Autodesk Inventor part; units mm, degrees
ref_plane "C1_XY" through (0, 0, 0) normal (0, 0, 1) x (1, 0, 0)
ref_plane "C1_YZ" through (0, 0, 0) normal (1, 0, 0) x (0, 1, 0)
ref_plane "C1_ZX" through (0, 0, 0) normal (0, 1, 0) x (0, 0, 1)
sketch "Sketch_1" plane through (0, 0, 0) normal (0, 0, 1) x (1, 0, 0)
  line L0 (-15, -4) -> (-15, -13)
  arc A0 (-15, -13) -> (-13, -15) centre (-13, -13) ccw
  line L1 (-13, -15) -> (-4, -15)
  line L2 (-4, -15) -> (-4, -13)
  line L3 (-4, -13) -> (-8.25, -13)
  line L4 (-8.25, -13) -> (-8.25, -9.6642)
  line L5 (-8.25, -9.6642) -> (-4.5858, -6)
  line L6 (-4.5858, -6) -> (-0.5196, -6)
  line L7 (-0.5196, -6) -> (0, -5.7)
  line L8 (0, -5.7) -> (0.5196, -6)
  line L9 (0.5196, -6) -> (4.5858, -6)
  line L10 (4.5858, -6) -> (8.25, -9.6642)
  line L11 (8.25, -9.6642) -> (8.25, -13)
  line L12 (8.25, -13) -> (4, -13)
  line L13 (4, -13) -> (4, -15)
  line L14 (4, -15) -> (13, -15)
  arc A1 (13, -15) -> (15, -13) centre (13, -13) ccw
  line L15 (15, -13) -> (15, -4)
  line L16 (15, -4) -> (13, -4)
  line L17 (13, -4) -> (13, -8.25)
  line L18 (13, -8.25) -> (9.6642, -8.25)
  line L19 (9.6642, -8.25) -> (6, -4.5858)
  line L20 (6, -4.5858) -> (6, -0.5196)
  line L21 (6, -0.5196) -> (5.7, 0)
  line L22 (5.7, 0) -> (6, 0.5196)
  line L23 (6, 0.5196) -> (6, 4.5858)
  line L24 (6, 4.5858) -> (9.6642, 8.25)
  line L25 (9.6642, 8.25) -> (13, 8.25)
  line L26 (13, 8.25) -> (13, 4)
  line L27 (13, 4) -> (15, 4)
  line L28 (15, 4) -> (15, 13)
  arc A2 (15, 13) -> (13, 15) centre (13, 13) ccw
  line L29 (13, 15) -> (4, 15)
  line L30 (4, 15) -> (4, 13)
  line L31 (4, 13) -> (8.25, 13)
  line L32 (8.25, 13) -> (8.25, 9.6642)
  line L33 (8.25, 9.6642) -> (4.5858, 6)
  line L34 (4.5858, 6) -> (0.5196, 6)
  line L35 (0.5196, 6) -> (0, 5.7)
  line L36 (0, 5.7) -> (-0.5196, 6)
  line L37 (-0.5196, 6) -> (-4.5858, 6)
  line L38 (-4.5858, 6) -> (-8.25, 9.6642)
  line L39 (-8.25, 9.6642) -> (-8.25, 13)
  line L40 (-8.25, 13) -> (-4, 13)
  line L41 (-4, 13) -> (-4, 15)
  line L42 (-4, 15) -> (-13, 15)
  arc A3 (-13, 15) -> (-15, 13) centre (-13, 13) ccw
  line L43 (-15, 13) -> (-15, 4)
  line L44 (-15, 4) -> (-13, 4)
  line L45 (-13, 4) -> (-13, 8.25)
  line L46 (-13, 8.25) -> (-9.6642, 8.25)
  line L47 (-9.6642, 8.25) -> (-6, 4.5858)
  line L48 (-6, 4.5858) -> (-6, 0.5196)
  line L49 (-6, 0.5196) -> (-5.7, 0)
  line L50 (-5.7, 0) -> (-6, -0.5196)
  line L51 (-6, -0.5196) -> (-6, -4.5858)
  line L52 (-6, -4.5858) -> (-9.6642, -8.25)
  line L53 (-9.6642, -8.25) -> (-13, -8.25)
  line L54 (-13, -8.25) -> (-13, -4)
  line L55 (-13, -4) -> (-15, -4)
extrude "Extrusion1" add sketch "Sketch_1" against normal blind 1440
sketch "Sketch2" plane through (0, 0, -1440) normal (0, 0, -1) x (-1, 0, 0)
  point P0 (0, 0)
hole "Hole1" at (0, 0, -1440) direction (0, 0, 1) diameter 6.8 depth 1440
sketch "Sketch3" plane through (0, 0, -1440) normal (0, 0, -1) x (-1, 0, 0)
  point P0 (-11.6, 11.6)
hole "Hole2" at (11.6, 11.6, -1440) direction (0, 0, 1) diameter 4.2 depth 1440
pattern_linear "Rectangular Pattern1" count 2 spacing 23.2 along (-1, 0, 0) count 2 spacing 23.2 along (0, -1, 0) of "Hole2"
ref_plane "C1_XY" through (0, 0, 0) normal (0, 0, 1) x (1, 0, 0)
ref_plane "C1_YZ" through (0, 0, 0) normal (1, 0, 0) x (0, 1, 0)
ref_plane "C1_ZX" through (0, 0, 0) normal (0, 1, 0) x (0, 0, 1)
ref_plane "to_frame_cap1_XY" through (0, 0, 0) normal (0, 0, 1) x (1, 0, 0)
ref_plane "to_frame_cap1_YZ" through (0, 0, 0) normal (1, 0, 0) x (0, 1, 0)
ref_plane "to_frame_cap1_ZX" through (0, 0, 0) normal (0, 1, 0) x (0, 0, 1)
ref_plane "to_frame_cap2_XY" through (0, 0, -1440) normal (0, 0, -1) x (1, 0, 0)
ref_plane "to_frame_cap2_YZ" through (0, 0, -1440) normal (1, 0, 0) x (0, -1, 0)
ref_plane "to_frame_cap2_ZX" through (0, 0, -1440) normal (0, -1, 0) x (0, 0, -1)
properties part number "HFS6-3030-1440"
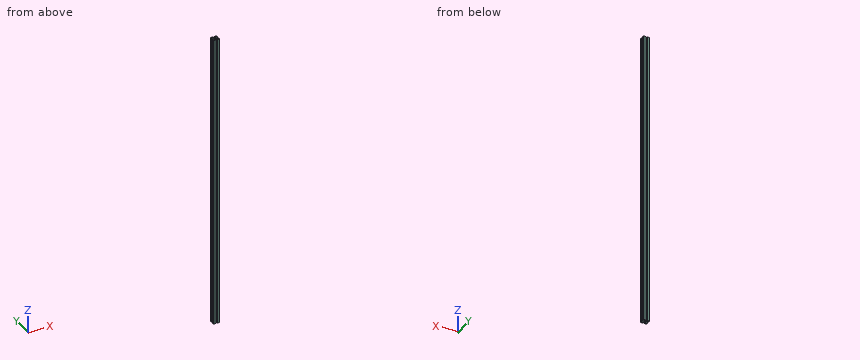
CAD build for the part. Positions are in the model's coordinates, mm. Coordinates: 2 decimals unless noted, no trailing zeros. Write item = value, one per line. Start each with the question number.
Q1. Flat gauge pins, fed straight in: pin 1 Ø1 at (y, z) = (-2.5, -643) entering from +X; pin 2 Ø1 at (y, z) = (-2, -748) entering from -X; pin 3 Ø1 at (x, z) = (2.5, -1115.5) entering from -Y. Where does each tip first touch, or does it go through?
Q2. Cut at A-A, the plane z = -923. Give the number of separate pieces and of enclosed holes in the cut face, then the cut area to 3 significant figures.
Q3. Drill centre lines: L1, parallel to Y at x = 11.6, z = -830; L2, parallel to Y at x = 12.25, z = -227. Where is each one in solid material? Low to high.
Computed:
q1.pin_1 = 6
q1.pin_2 = -6
q1.pin_3 = -6
q2.separate_pieces = 1
q2.enclosed_holes = 5
q2.area = 332 mm²
q3.L1 = -15 to -13.7, -9.5 to -8.25, 8.25 to 9.5, 13.7 to 15
q3.L2 = -15 to -13.6, -9.6 to -8.25, 8.25 to 9.6, 13.6 to 15
